Build history of the part. All positions in model axes, mm. Round coordinates to 2 decimals unless told otherwise and drop trailing zeros. Write each loop counter-clockwise with the first axis right and the second up, starting at its lowest first coordinate (ties: lowest second). Pieces come first, ordered by that corner, then holes. Notation, with made-up numbers: (36.25, -17) -> (91.25, -17) arc R32 ccw to (91.25, 9) -> close; hole circle Ø11 at (-36, 80). An arc over 180 degrees is marked (long way). One line per question, with ' | ' between items.
from build123d import *

# Parameters (mm, degrees)
SKETCH1_R           = 1.5
SKETCH1_R_2         = 13.9
BOSS_EXTRUDE1_DEPTH = 3


with BuildPart() as part:
    # Sketch1 → Boss-Extrude1 (new body)
    with BuildSketch(Plane(origin=(0, 0, 0), x_dir=(1, 0, 0), z_dir=(0, 1, 0))):
        with BuildLine():
            Line((3.491378029, 30.5), (-3.491378029, 30.5))
            ThreePointArc((-3.491378029, 30.5), (-5.40479519, 30.119397663), (-7.026911935, 29.035533906))
            Line((-7.026911935, 29.035533906), (-29.035533906, 7.026911935))
            ThreePointArc((-29.035533906, 7.026911935), (-30.119397663, 5.40479519), (-30.5, 3.491378029))
            Line((-30.5, 3.491378029), (-30.5, -3.491378029))
            ThreePointArc((-30.5, -3.491378029), (-30.119397663, -5.40479519), (-29.035533906, -7.026911935))
            Line((-29.035533906, -7.026911935), (-7.026911935, -29.035533906))
            ThreePointArc((-7.026911935, -29.035533906), (-5.40479519, -30.119397663), (-3.491378029, -30.5))
            Line((-3.491378029, -30.5), (3.491378029, -30.5))
            ThreePointArc((3.491378029, -30.5), (5.40479519, -30.119397663), (7.026911935, -29.035533906))
            Line((7.026911935, -29.035533906), (29.035533906, -7.026911935))
            ThreePointArc((29.035533906, -7.026911935), (30.119397663, -5.40479519), (30.5, -3.491378029))
            Line((30.5, -3.491378029), (30.5, 3.491378029))
            ThreePointArc((30.5, 3.491378029), (30.119397663, 5.40479519), (29.035533906, 7.026911935))
            Line((29.035533906, 7.026911935), (7.026911935, 29.035533906))
            ThreePointArc((7.026911935, 29.035533906), (5.40479519, 30.119397663), (3.491378029, 30.5))
        make_face()
        with Locations((-8.131727984, -22.273863607)):
            Circle(SKETCH1_R, mode=Mode.SUBTRACT)
        with Locations((8.131727984, -22.273863607)):
            Circle(SKETCH1_R, mode=Mode.SUBTRACT)
        with Locations((22.273863607, -8.131727984)):
            Circle(SKETCH1_R, mode=Mode.SUBTRACT)
        with Locations((22.273863607, 8.131727984)):
            Circle(SKETCH1_R, mode=Mode.SUBTRACT)
        with Locations((8.131727984, 22.273863607)):
            Circle(SKETCH1_R, mode=Mode.SUBTRACT)
        with Locations((-8.131727984, 22.273863607)):
            Circle(SKETCH1_R, mode=Mode.SUBTRACT)
        with Locations((-22.273863607, -8.131727984)):
            Circle(SKETCH1_R, mode=Mode.SUBTRACT)
        with Locations((-22.273863607, 8.131727984)):
            Circle(SKETCH1_R, mode=Mode.SUBTRACT)
        Circle(SKETCH1_R_2, mode=Mode.SUBTRACT)
    extrude(amount=BOSS_EXTRUDE1_DEPTH)


solid = part.part
(1) Slice it at C-C (y = 1.5). State how many separate pieces and enclosed holes the cut face has, then the cut area to 3 significant figures.
Calculated:
separate pieces: 1 | enclosed holes: 9 | area: 1,810 mm2
(2) Slice it at B-B (z = 0). Write the cut outline in (x, y), then the cut area to 3 significant figures.
Calculated:
outline: (-30.5, 0) -> (-13.9, 0) -> (-13.9, 3) -> (-30.5, 3) -> close; (13.9, 0) -> (30.5, 0) -> (30.5, 3) -> (13.9, 3) -> close | area: 99.6 mm2
(3) Drop flat-ended pins along their axis: pin 1 (5 mm diameter, centred on x = 8.13, z = 22.27, fed in from +Y); pin 2 (1 mm diameter, centred on x = -16.5, y = 2, fed in from -Z); pin 3 (1.5 mm diameter, centred on x = 18, y = 0.5, fed in from -Z). Give the stop position or say it passes through.
Calculated:
pin 1: y = 3 | pin 2: z = -20.06 | pin 3: z = -18.81
(4) Slice it at D-D (z = 15). Write the cut outline in (x, y).
Calculated:
outline: (-21.06, 0) -> (21.06, 0) -> (21.06, 3) -> (-21.06, 3) -> close
(5) Wall check: line 1 (Z direction, x = -7, y = 1.25); line 2 (Z direction, x = -8, y = 1.2); line 3 (X direction, y = 1.8, z = -9.5). Give the ranges that are in metal, low to high. Write a range as from..to.
Calculated:
line 1: -29.06..-23.26, -21.29..-12.01, 12.01..21.29, 23.26..29.06 | line 2: -28.06..-23.77, -20.78..-11.37, 11.37..20.78, 23.77..28.06 | line 3: -26.56..-22.89, -21.66..-10.15, 10.15..21.66, 22.89..26.56
(6) Slice it at A-A (x = 0). Write the cut outline in (y, z), then the cut area to 3 significant figures.
Calculated:
outline: (0, -30.5) -> (3, -30.5) -> (3, -13.9) -> (0, -13.9) -> close; (0, 13.9) -> (3, 13.9) -> (3, 30.5) -> (0, 30.5) -> close | area: 99.6 mm2
(7) Mould opens along Z. For faces 1 (the cylindrical face through (-23.464, 1.479, 9.044)), 2 (the flat face through (-14, 3, -7)), 3 (the flat face through (0, 1, 30.5)) say: pulls with the +Z half, pulls with the -Z half, needs draft (parallel to the pull), parting line crosses it, or undercut.
Calculated:
face 1: undercut | face 2: needs draft | face 3: pulls with the +Z half
